from build123d import *

# Parameters (mm, degrees)
EXTRUDE_1_DEPTH     = 30
CHAMFER_2_SIZE      = 5
SKETCH_2_R          = 2.6
CUT_EXTRUDE_1_DEPTH = 127.194294641
SKETCH_3_W          = 10
SKETCH_3_H          = 15
CUT_EXTRUDE_2_DEPTH = 107.301458127
SKETCH_4_R          = 2.6
CUT_EXTRUDE_3_DEPTH = 126.299640861
FILLET_1_R          = 1.5


with BuildPart() as part:
    # 草图1 → 凸台-拉伸1 (new body)
    with BuildSketch(Plane.XY):
        Polygon((20, 0), (20, -20), (40, -20), (40, -5), (80, -5), (80, -20), (100, -20), (100, 0), (120, 0), (120, 5), (0, 5), (0, 0), align=None)
    extrude(amount=EXTRUDE_1_DEPTH)

    # 倒角2
    chamfer_2_edges = [part.edges().sort_by_distance(p)[0] for p in [
        (80, -5, 15),
        (40, -5, 15),
    ]]
    chamfer(chamfer_2_edges, length=CHAMFER_2_SIZE)

    # 草图2 → 切除-拉伸1 (cut, through all)
    with BuildSketch(Plane(origin=(0, 5, 0), x_dir=(1, 0, 0), z_dir=(0, 1, 0))):
        with Locations(Location((10, -7.5, 0), (0, 0, 270))):
            Circle(SKETCH_2_R)
        with Locations(Location((10, -22.5, 0), (0, 0, 270))):
            Circle(SKETCH_2_R)
        with Locations(Location((110, -22.5, 0), (0, 0, 270))):
            Circle(SKETCH_2_R)
        with Locations(Location((110, -7.5, 0), (0, 0, 270))):
            Circle(SKETCH_2_R)
    extrude(amount=-CUT_EXTRUDE_1_DEPTH, mode=Mode.SUBTRACT)

    # 草图3 → 切除-拉伸2 (cut, through all)
    with BuildSketch(Plane.ZY.offset(-20)):
        with Locations((15, -12.5)):
            Rectangle(SKETCH_3_W, SKETCH_3_H)
    extrude(amount=-CUT_EXTRUDE_2_DEPTH, mode=Mode.SUBTRACT)

    # 草图4 → 切除-拉伸3 (cut, through all)
    with BuildSketch(Plane(origin=(0, 0, 0), x_dir=(-1, 0, 0), z_dir=(0, 0, -1))):
        with Locations((-87.5, -12.5)):
            Circle(SKETCH_4_R)
        with Locations((-32.5, -12.5)):
            Circle(SKETCH_4_R)
    extrude(amount=-CUT_EXTRUDE_3_DEPTH, mode=Mode.SUBTRACT)

    # 圆角1
    fillet_1_edges = [part.edges().sort_by_distance(p)[0] for p in [
        (20, 0, 15),
        (100, 0, 15),
    ]]
    fillet(fillet_1_edges, radius=FILLET_1_R)


solid = part.part
Check sheet for the modelled part. Datum: model origin and axes. Units: mm. A direction names the side the tool comes from. Round coordinates to 2 decimals unless told otherwise and drop trailing zeros. Loops run counter-clockwise (first coordinate to the right, second up) from the corner with the lowest first, then second, coordinate; pieces in that order, holes last. Notation, with made-up numbers: (-40, 11) -> (4, 11) arc R30 ccw to (4, 39) -> close; hole circle Ø11 at (54, 8). An arc over 180 degrees is marked (long way). Put each result on its own line as item: value. Start each with the question number.
1. Access from +Z, -Z, +X, -X, +Y, -Y to the whole of each face (thin tool, end or side, straight path). Record for faces 1 (the face through (78, -8, 25)), 2 (the face through (90, -11, 10)), 3 (the face through (111, 0, 15)), 4 (the face through (20, -4, 15)).
2. Section check D-D (y = -12.5). Give the number of separate pieces and of enclosed holes in the cut face, plus the area to 3 significant figures.
3. Section check B-B (y = -17.25). Enter the section's corners in (x, z).
4. Gauge pin test, flat ends, axial feed: pin 1 (5 mm diameter, centred on y = -15, z = 3, fed in from +X); pin 2 (9 mm diameter, centred on x = 114.5, z = 21.5, fed in from -Y); pin 3 (8 mm diameter, centred on y = -13, z = 24.5, fed in from -X). Record the tip position at first contact, or that the pin passes through.
5. Draft check along Y on faces 5 (the face through (90.1, -12.4, 24.9)), 6 (the face through (40, -15, 25)), 7 (the face through (43, -7, 25)). Enter one of: +Y half, -Y half, draft (parallel to the pull), parting line (faces both ways), or undercut.
6. Section check A-A (x = 10). Enter the section's corners in (y, z).
7. Section check C-C (z = 22.5). Enter the section's corners in (x, y), plus the area to 3 significant figures.
8. Scan lines: probe 1 along X at (y, z) = (3, 22.5); probe 2 along Y at (x, z) = (32.5, 6); probe 3 along X at (y, z) = (-16.25, 23). Record each from-to range of solid material in increasing order.
Findings:
1. face 1: +Z, -Z, -Y
1. face 2: +X, -X, -Y
1. face 3: +Z, -Z, +X, -Y
1. face 4: +Z, -Z, -X, -Y
2. separate pieces: 8
2. enclosed holes: 0
2. area: 592 mm^2
3. outline: (20, 0) -> (40, 0) -> (40, 10) -> (20, 10) -> close; (20, 20) -> (40, 20) -> (40, 30) -> (20, 30) -> close; (80, 0) -> (100, 0) -> (100, 10) -> (80, 10) -> close; (80, 20) -> (100, 20) -> (100, 30) -> (80, 30) -> close
4. pin 1: stops at x = 100
4. pin 2: stops at y = 0
4. pin 3: stops at x = 20
5. face 5: undercut
5. face 6: draft
5. face 7: -Y half
6. outline: (0, 0) -> (5, 0) -> (5, 4.9) -> (0, 4.9) -> close; (0, 10.1) -> (5, 10.1) -> (5, 19.9) -> (0, 19.9) -> close; (0, 25.1) -> (5, 25.1) -> (5, 30) -> (0, 30) -> close
7. outline: (0, 0) -> (7.4, 0) -> (7.4, 5) -> (0, 5) -> close; (12.6, 0) -> (18.5, 0) arc R1.5 cw to (20, -1.5) -> (20, -20) -> (40, -20) -> (40, -10) -> (45, -5) -> (75, -5) -> (80, -10) -> (80, -20) -> (100, -20) -> (100, -1.5) arc R1.5 cw to (101.5, 0) -> (107.4, 0) -> (107.4, 5) -> (12.6, 5) -> close; (112.6, 0) -> (120, 0) -> (120, 5) -> (112.6, 5) -> close; hole circle Ø5.2 at (32.5, -12.5); hole circle Ø5.2 at (87.5, -12.5)
7. area: 1,530 mm^2
8. probe 1: x = 0 to 7.4, 12.6 to 107.4, 112.6 to 120
8. probe 2: y = -20 to -15.1, -9.9 to 5
8. probe 3: x = 20 to 40, 80 to 100
